Autodesk Inventor part; units mm, degrees
ref_plane "YZ Plane" through (0, 0, 0) normal (1, 0, 0) x (0, 1, 0)
ref_plane "XZ Plane" through (0, 0, 0) normal (0, 1, 0) x (-1, 0, 0)
ref_plane "XY Plane" through (0, 0, 0) normal (0, 0, 1) x (1, 0, 0)
sketch "Skizze1" plane through (0, 0, 0) normal (0, 0, 1) x (1, 0, 0)
  line L0 (0, 0) -> (526.5, 0)
  line L1 (526.5, 0) -> (526.5, 72.5)
  line L2 (526.5, 72.5) -> (0, 72.5)
  line L3 (0, 72.5) -> (0, 0)
  line L4 (0, 72.5) -> (35, 72.5)
  line L5 (35, 72.5) -> (35, 66.15)
  line L6 (35, 66.15) -> (0, 66.15)
  line L7 (0, 66.15) -> (0, 72.5)
  line L8 (0, 72.5) -> (6.35, 72.5)
  line L9 (6.35, 72.5) -> (6.35, 37.5)
  line L10 (6.35, 37.5) -> (0, 37.5)
  line L11 (0, 37.5) -> (0, 72.5)
  line L12 (0, 36.25) -> (526.5, 36.25) construction
  line L13 (263.25, 72.5) -> (263.25, 0) construction
  line L14 (0, 0) -> (35, 0)
  line L15 (35, 0) -> (35, 6.35)
  line L16 (35, 6.35) -> (0, 6.35)
  line L17 (0, 6.35) -> (0, 0)
  line L18 (0, 0) -> (6.35, 0)
  line L19 (6.35, 0) -> (6.35, 35)
  line L20 (6.35, 35) -> (0, 35)
  line L21 (0, 35) -> (0, 0)
  line L22 (526.5, 72.5) -> (526.5, 0)
  line L23 (526.5, 72.5) -> (491.5, 72.5)
  line L24 (491.5, 72.5) -> (491.5, 66.15)
  line L25 (491.5, 66.15) -> (526.5, 66.15)
  line L26 (526.5, 66.15) -> (526.5, 72.5)
  line L27 (526.5, 72.5) -> (520.15, 72.5)
  line L28 (520.15, 72.5) -> (520.15, 37.5)
  line L29 (520.15, 37.5) -> (526.5, 37.5)
  line L30 (526.5, 37.5) -> (526.5, 72.5)
  line L31 (526.5, 0) -> (520.15, 0)
  line L32 (526.5, 0) -> (491.5, 0)
  line L33 (491.5, 0) -> (491.5, 6.35)
  line L34 (491.5, 6.35) -> (526.5, 6.35)
  line L35 (520.15, 0) -> (520.15, 35)
  line L36 (526.5, 6.35) -> (526.5, 0)
  line L37 (520.15, 35) -> (526.5, 35)
  line L38 (526.5, 35) -> (526.5, 0)
  point P0 (526.5, 37.5)
  point P1 (520.15, 66.15)
  point P2 (6.35, 66.15)
  point P3 (0, 37.5)
  point P4 (0, 35)
  point P5 (6.35, 6.35)
  point P6 (491.5, 0)
  point P7 (520.15, 6.35)
  point P8 (526.5, 35)
  dimension "d0" = 526.5
  dimension "d1" = 72.5
  dimension "d2" = 35
  dimension "d3" = 6.35
  dimension "d4" = 6.35
  dimension "d5" = 35
extrude "Extrusion1" add sketch "Skizze1" along normal blind 4 contours L15 L16 L19 L20 L3 L10 L9 L6 L5 L2 L24 L25 L28 L29 L1 L37 L35 L34 L33 L0
properties part number "103.012.01_Abdeckung_Gestell_front" material "PMMA-Kunststoff"
Geometry: final body of the model. Coordinates: model frame, mm. Round coordinates to 2 decimals unless told otherwise and drop trailing zeros. Write each loop counter-clockwise with the first axis right and the second up, starting at its lowest first coordinate (ties: lowest second). Pieces come first, ordered by that corner, then holes.
Item 1: Pin query (flat end, axial travel): P1, Ø4, axis at x = 260, y = 17.5, coming from the -Z side; P2, Ø1.2, axis at x = 1.5, z = 3, coming from the +Y side; P3, Ø2, axis at y = 8, z = 3.5, coming from the -X side; P4, Ø2, axis at y = 9, z = 3, coming from the +X side. Return the tip coordinate at first contact, or that it passes through.
Item 2: Material intervals for L1, parallel to X at y = 44, z = 3.6; L2, parallel to X at y = 67.5, z = 2.05; L3, parallel to Y at x = 23.5, z = 2.6, sorted ascending.
Item 3: Section query B-B (y = 24). Return loops of the section in (x, z).
Item 4: Section query A-A (z = 3.2). Return loops of the section in (x, y).
Completed:
1. P1: stops at z = 0
1. P2: stops at y = 37.5
1. P3: stops at x = 6.35
1. P4: stops at x = 520.15
2. L1: x = 6.35 to 520.15
2. L2: x = 35 to 491.5
2. L3: y = 6.35 to 66.15
3. outline: (6.35, 0) - (520.15, 0) - (520.15, 4) - (6.35, 4) - close
4. outline: (0, 35) - (6.35, 35) - (6.35, 6.35) - (35, 6.35) - (35, 0) - (491.5, 0) - (491.5, 6.35) - (520.15, 6.35) - (520.15, 35) - (526.5, 35) - (526.5, 37.5) - (520.15, 37.5) - (520.15, 66.15) - (491.5, 66.15) - (491.5, 72.5) - (35, 72.5) - (35, 66.15) - (6.35, 66.15) - (6.35, 37.5) - (0, 37.5) - close
